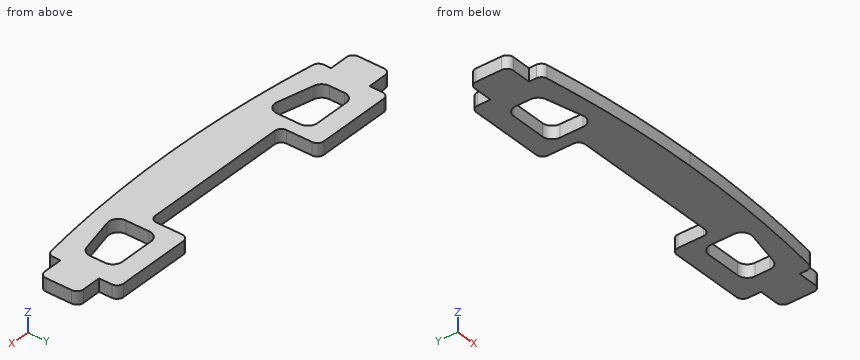
```python
from build123d import *

# Parameters (mm, degrees)
RESSALTO_EXTRUS_O1_DEPTH = 2


with BuildPart() as part:
    # Esboço1 → Ressalto-extrusão1 (new body)
    with BuildSketch(Plane.XY):
        with BuildLine():
            Line((-11.5, 0), (11.5, 0))
            ThreePointArc((11.5, 0), (12.207106781, 0.292893219), (12.5, 1))
            Line((12.5, 1), (12.5, 5))
            ThreePointArc((12.5, 5), (12.792893219, 5.707106781), (13.5, 6))
            Line((13.5, 6), (25, 6))
            ThreePointArc((25, 6), (25.707106781, 5.707106781), (26, 5))
            Line((26, 5), (26, 3))
            Line((26, 3), (29, 3))
            ThreePointArc((29, 3), (29.707106781, 2.707106781), (30, 2))
            Line((30, 2), (30, -2))
            ThreePointArc((30, -2), (29.707106781, -2.707106781), (29, -3))
            Line((29, -3), (26, -3))
            Line((26, -3), (26, -4.140659326))
            ThreePointArc((26, -4.140659326), (25.757604446, -4.793373278), (25.147928994, -5.12965731))
            ThreePointArc((25.147928994, -5.12965731), (12.608692582, -6.531769505), (0, -7))
            ThreePointArc((0, -7), (-12.608692582, -6.531769505), (-25.147928994, -5.12965731))
            ThreePointArc((-25.147928994, -5.12965731), (-25.757604446, -4.793373278), (-26, -4.140659326))
            Line((-26, -4.140659326), (-26, -3))
            Line((-26, -3), (-29, -3))
            ThreePointArc((-29, -3), (-29.707106781, -2.707106781), (-30, -2))
            Line((-30, -2), (-30, 2))
            ThreePointArc((-30, 2), (-29.707106781, 2.707106781), (-29, 3))
            Line((-29, 3), (-26, 3))
            Line((-26, 3), (-26, 5))
            ThreePointArc((-26, 5), (-25.707106781, 5.707106781), (-25, 6))
            Line((-25, 6), (-13.5, 6))
            ThreePointArc((-13.5, 6), (-12.792893219, 5.707106781), (-12.5, 5))
            Line((-12.5, 5), (-12.5, 1))
            ThreePointArc((-12.5, 1), (-12.207106781, 0.292893219), (-11.5, 0))
        make_face()
        with BuildLine():
            Line((15.99403097, 3), (21.50596903, 3))
            ThreePointArc((21.50596903, 3), (22.56240846, 2.56240846), (23, 1.50596903))
            Line((23, 1.50596903), (23, -0.816705571))
            ThreePointArc((23, -0.816705571), (22.677159402, -1.744305514), (21.848160888, -2.271020968))
            Line((21.848160888, -2.271020968), (16.336222828, -3.56794757))
            ThreePointArc((16.336222828, -3.56794757), (15.066431028, -3.284822545), (14.5, -2.113632174))
            Line((14.5, -2.113632174), (14.5, 1.50596903))
            ThreePointArc((14.5, 1.50596903), (14.93759154, 2.56240846), (15.99403097, 3))
        make_face(mode=Mode.SUBTRACT)
        with BuildLine():
            Line((-14.5, -2.113632174), (-14.5, 1.50596903))
            ThreePointArc((-14.5, 1.50596903), (-14.93759154, 2.56240846), (-15.99403097, 3))
            Line((-15.99403097, 3), (-21.50596903, 3))
            ThreePointArc((-21.50596903, 3), (-22.56240846, 2.56240846), (-23, 1.50596903))
            Line((-23, 1.50596903), (-23, -0.816705571))
            ThreePointArc((-23, -0.816705571), (-22.677159402, -1.744305514), (-21.848160888, -2.271020968))
            Line((-21.848160888, -2.271020968), (-16.336222828, -3.56794757))
            ThreePointArc((-16.336222828, -3.56794757), (-15.066431028, -3.284822545), (-14.5, -2.113632174))
        make_face(mode=Mode.SUBTRACT)
    extrude(amount=RESSALTO_EXTRUS_O1_DEPTH)


solid = part.part
```
Input: part model. Units: mm. Frame: model coordinates. Coordinates: 2 decimals unless noted, no trailing zeros. Loops run counter-clockwise (first coordinate to the right, second up) from the corner with the lowest first, then second, coordinate; pieces in that order, holes last. Notation, with made-up numbers: M 77,-20.5 L 109,-20.5 A23 ccw 109,18.5 Z; hole C -7,67.25 d3. An arc over 180 degrees is marked long. Use a Markdown table: item, result. Add a question column.
1) Pin query (flat end, axial travel): P1, Ø0.6, axis at x = 19, z = 1, coming from the -Y side; P2, Ø6, axis at x = 23, y = 1, coming from the -Z side; P3, Ø0.6, axis at x = 5.5, z = 1.5, coming from the +Y side; P4, Ø1, axis at x = 27.5, z = 0.5, coming from the +Y side. Return the tip coordinate at first contact, or that it passes through.
2) Section B-B, the plane x = -15.5. Return the cut outline in (y, z).
3) Section A-A, the plane y = 4.5. Return the cut outline in (x, z).
4) Section D-D, the plane x = 4. Return the cut outline in (y, z), plus the area to 3 significant figures.
5) Line query: L1, parallel to X at y = -0.25, z = 0.5; L2, parallel to X at y = 4.25, z = 0.35; L3, parallel to X at y = 2, z = 0.85. Output: solid intervals per line, ascending. Write a range as from..to.
6) Section C-C, the plane z = 0.35. Give the number of separate pieces and of enclosed holes in the cut face, plus the area to 3 significant figures.
Answer below:
| question | item | result |
|---|---|---|
| 1 | P1 | y = -5.97 |
| 1 | P2 | z = 0 |
| 1 | P3 | y = 0 |
| 1 | P4 | y = 3 |
| 2 | outline | M -6.29,0 L -3.52,0 L -3.52,2 L -6.29,2 Z; M 2.92,0 L 6,0 L 6,2 L 2.92,2 Z |
| 3 | outline | M -26,0 L -12.5,0 L -12.5,2 L -26,2 Z; M 12.5,0 L 26,0 L 26,2 L 12.5,2 Z |
| 4 | outline | M -6.95,0 L 0,0 L 0,2 L -6.95,2 Z |
| 4 | area | 13.9 mm2 |
| 5 | L1 | -30..-23, -14.5..14.5, 23..30 |
| 5 | L2 | -26..-12.5, 12.5..26 |
| 5 | L3 | -30..-22.92, -14.58..-12.5, 12.5..14.58, 22.92..30 |
| 6 | separate pieces | 1 |
| 6 | enclosed holes | 2 |
| 6 | area | 440 mm2 |
